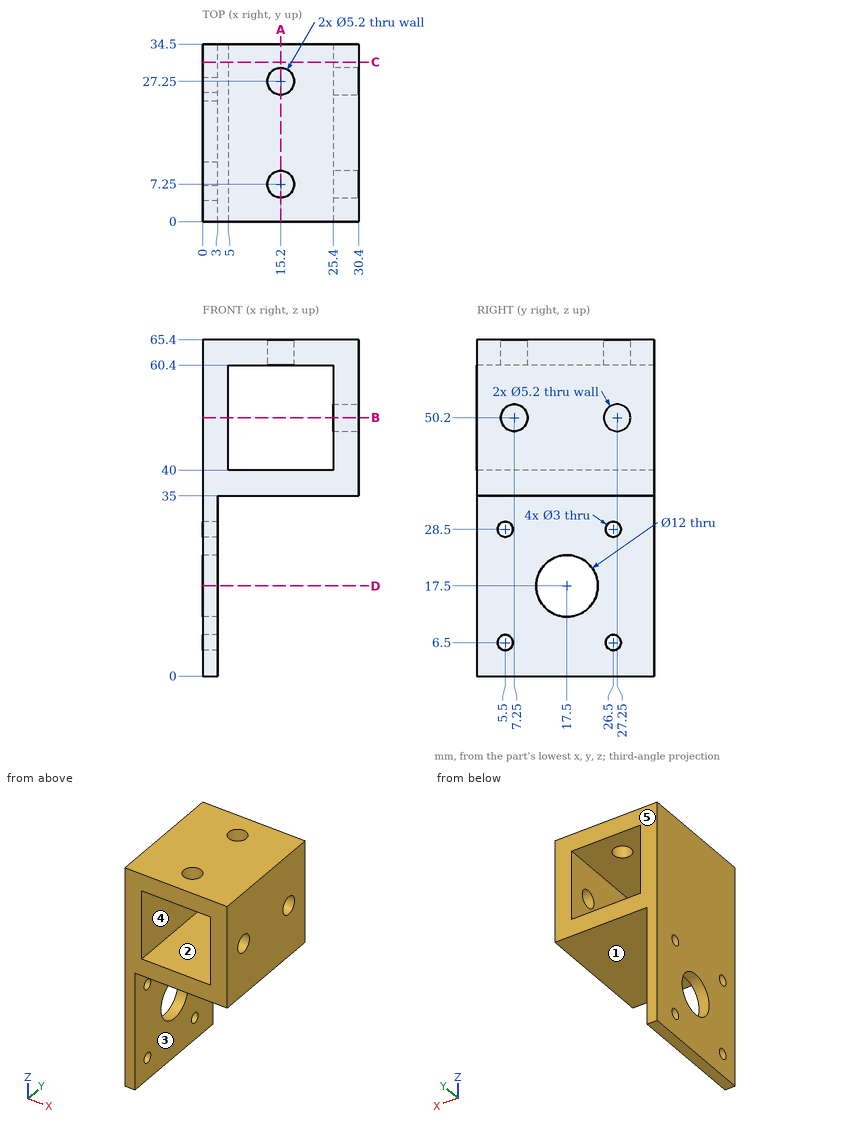
Drawing for the job (mm, zero at the part's lowest x, y, z). A direction names the side the tool comes from. Give positions to 0.01 mm unless a question says otherwise; leave off trailing zeros. Order: outer loops, then holes, each group sorted by start corner. A loop starts at its lowest first (then second) coordinate and runs counter-clockwise, first axis right, second up. Notation, with made-up numbers: M -6,53 L 22,53 A28 cw 22,82 Z; hole C -27,3.5 d11. An arc over 180 degrees is marked long. Write item = value, one per line. Start each with the question number.
(1) Slice it at C-C on y = 31. Write the cut outline in (x, z).
(2) Two-plate mould, pull along X, no slides. Class the marked faces 1, 2 and 3: released by +X, released by -X, zero draft, split by the parting line, or undercut.
(3) Slice it at B-B on z = 50.2. Write the cut outline in (x, y), plus the area to 3 significant figures.
(4) Pin check, flat tips, straight feed: pin 1 Ø2.5 at (y, z) = (26.5, 28.5) entering from +X; pin 2 Ø10 at (x, y) = (15.5, 18.5) entering from -Z; pin 3 Ø19 at (y, z) = (17.5, 17.5) entering from +X; pin 4 Ø4.5 at (y, z) = (27.25, 50.2) entering from +X. Stop position of each tip, or through.
(5) Slice it at D-D on z = 17.5. Write the cut outline in (x, y).
(6) Which spindle directions (+Z, -Z, +X, -X, +Y, -Y) get a long thin tool onto all of the face, cutting with end or side? Do the marked faces 4 and 5. Say none if no direction does.
(7) Slice it at A-A on x = 15.2. Write the cut outline in (y, z), plus the area to 3 significant figures.
(8) Probe L1, parallel to Y at x = 15.2, z = 61.5; L2, parallel to Z at x = 2.2, y = 5.5; L3, parallel to Z at x = 9, y = 8. List the from-to ranges inside material, lowest first. Write a range as [from, to].
Responses:
q1.outline = M 0,0 L 3,0 L 3,35 L 30.4,35 L 30.4,65.4 L 0,65.4 Z; hole M 5,40 L 25.4,40 L 25.4,60.4 L 5,60.4 Z
q2.face_1 = zero draft
q2.face_2 = undercut
q2.face_3 = released by +X
q3.outline = M 0,0 L 5,0 L 5,34.5 L 0,34.5 Z; M 25.4,0 L 30.4,0 L 30.4,4.65 L 25.4,4.65 Z; M 25.4,9.85 L 30.4,9.85 L 30.4,24.65 L 25.4,24.65 Z; M 25.4,29.85 L 30.4,29.85 L 30.4,34.5 L 25.4,34.5 Z
q3.area = 293 mm2
q4.pin_1 = through
q4.pin_2 = 35
q4.pin_3 = 3
q4.pin_4 = 5
q5.outline = M 0,0 L 3,0 L 3,11.5 L 0,11.5 Z; M 0,23.5 L 3,23.5 L 3,34.5 L 0,34.5 Z
q6.face_4 = +Y, -Y
q6.face_5 = +Z, -Z, +X, -X, +Y
q7.outline = M 0,35 L 34.5,35 L 34.5,40 L 0,40 Z; M 0,60.4 L 4.65,60.4 L 4.65,65.4 L 0,65.4 Z; M 9.85,60.4 L 24.65,60.4 L 24.65,65.4 L 9.85,65.4 Z; M 29.85,60.4 L 34.5,60.4 L 34.5,65.4 L 29.85,65.4 Z
q7.area = 293 mm2
q8.L1 = [0, 4.65], [9.85, 24.65], [29.85, 34.5]
q8.L2 = [0, 5], [8, 27], [30, 65.4]
q8.L3 = [35, 40], [60.4, 65.4]
